Design review of the part shown in the three views and the two pictorial views. Dimensions are in mm from the part's minimum x, y and z. A direction names the side the tool comes from. Give positions to 0.01 mm unless a question says otherwise; leave off trailing zeros. Order: outer loops, then holes, each group sorted by start corner. A loop starts at its lowest first (then second) coordinate and runs counter-clockwise, first axis right, second up.
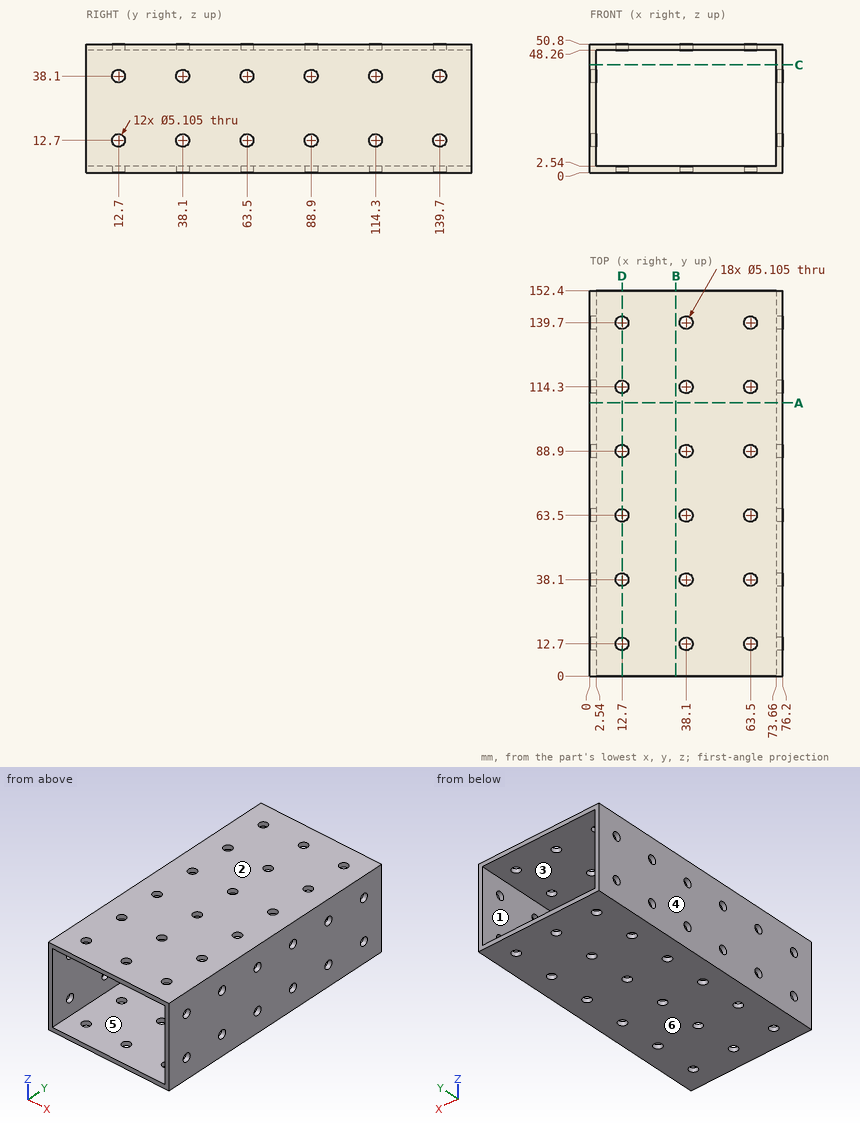
Item 1: For the marked faces 1 and 2, list the 3-axis set-ups (+Z, -Z, +X, -X, +Y, -Y) from which the entire face can be reached by the end or side of a thin tool; tool diameter is ignored.
Values found:
face 1: +Y, -Y
face 2: +Z, +X, -X, +Y, -Y
Item 2: Take a section at A-A (y = 108). Give the boundary of the cut face in (x, z).
Values found:
outline: (0, 0) - (76.2, 0) - (76.2, 50.8) - (0, 50.8) - close; hole (2.54, 2.54) - (73.66, 2.54) - (73.66, 48.26) - (2.54, 48.26) - close
Item 3: For line 1 (Z direction, x = 2, y = 88.9); line 2 (Z direction, x = 45, y = 65); line 3 (X direction, y = 88.5, z = 27), list the stretches that pass through material, from the lowest coordinate up.
Values found:
line 1: z = 0 to 10.15, 15.25 to 35.55, 40.65 to 50.8
line 2: z = 0 to 2.54, 48.26 to 50.8
line 3: x = 0 to 2.54, 73.66 to 76.2
Item 4: Take a section at B-B (x = 34). Give the boundary of the cut face in (y, z).
Values found:
outline: (0, 0) - (152.4, 0) - (152.4, 2.54) - (0, 2.54) - close; (0, 48.26) - (152.4, 48.26) - (152.4, 50.8) - (0, 50.8) - close
Item 5: Draft analysis for pull direction Z (two halves, no side actions). For the marked faces 3, 4, 5 and 6, state which applies: released by +Z, released by -Z, zero draft, split by the parting line, or undercut.
Values found:
face 3: undercut
face 4: zero draft
face 5: undercut
face 6: released by -Z
Item 6: Take a section at D-D (x = 12.7). Give the number of separate pieces and of enclosed holes in the cut face.
Values found:
separate pieces: 14
enclosed holes: 0
Item 7: Take a section at C-C (z = 42.5). Give the boundary of the cut face in (x, y).
Values found:
outline: (0, 0) - (2.54, 0) - (2.54, 152.4) - (0, 152.4) - close; (73.66, 0) - (76.2, 0) - (76.2, 152.4) - (73.66, 152.4) - close
